Check sheet for the modelled part. Datum: model origin and axes. Units: mm. Face numbers are marked on the shaded views. A direction names the side the tool comes from. Round coordinates to 2 decimals unless told otherwise and drop trailing zeros. Order: outer loops, then holes, each group sorted by start corner. A loop starts at its lowest first (then second) coordinate and runs counter-clockwise, first axis right, second up.
Q1. Cross-section at A-A on z = 9.5. Record the cut outline in (x, y), then the cut area to 3 significant figures.
Q2. Cross-section at B-B on x = 1.8. Record the cut outline in (y, z).
Q3. Cross-section at C-C on y = 8.25. Record the cut outline in (x, z).
Q4. Set-up check for the marked faces 5, 6, 7, 8 and 9: record each of +Z, -Z, +X, -X, +Y, -Y from which the full face is reachable in a straight line by a thin tool's end or side.
Q5. Mould release check, pull along Y, two halves, no side actions. Record for the marked faces 1, 2, 3 and 4: +Y half, -Y half, draft (parallel to the pull), parting line (faces both ways), or undercut.
Q6. Scan lines: probe 1 along Y at (x, z) = (1.9, 10); probe 2 along Z at (x, y) = (2.05, -5.25); probe 3 along Y at (x, z) = (0.2, -6.25). Record each from-to range of solid material in increasing order.
Q7. Depth check by flat-ended pin: P1, Ø1.2, axis at x = 1.5, y = -8.5, coming from the +Z side; P2, Ø0.8, axis at x = 1.5, z = -2, coming from the -Y side; P3, Ø0.8, axis at x = 1.5, y = 3, coming from the +Z side. Enter the tip coordinate at first touch or a pass-through.
from build123d import *

# Parameters (mm, degrees)
BOSS_EXTRUDE1_DEPTH = 2.5


with BuildPart() as part:
    # Sketch2 → Boss-Extrude1 (new body)
    with BuildSketch(Plane(origin=(0, 0, 0), x_dir=(0, 0, -1), z_dir=(1, 0, 0))):
        Polygon((-8.75, 11.25), (11.25, -3.75), (11.25, -6.25), (8.75, -6.25), (8.75, -11.25), (3.75, -11.25), (3.75, -6.25), (1.25, -6.25), (1.25, -3.75), (-11.25, -3.75), (-11.25, 1.25), (-8.75, 1.25), (-8.75, 6.25), (-11.25, 6.25), (-11.25, 11.25), align=None)
    extrude(amount=BOSS_EXTRUDE1_DEPTH)


solid = part.part
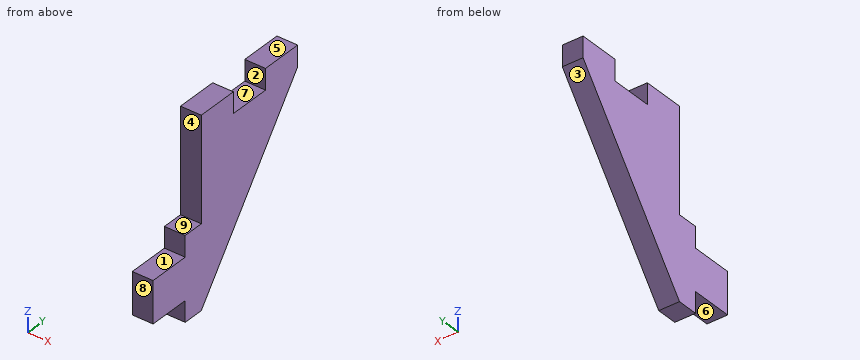
Results found:
1. outline: (0, -3.75) - (2.5, -3.75) - (2.5, 1.25) - (0, 1.25) - close; (0, 6.25) - (2.5, 6.25) - (2.5, 11.25) - (0, 11.25) - close
1. area: 25.0 mm2
2. outline: (-11.25, -8.75) - (-6.25, -8.75) - (-6.25, -11.25) - (-3.75, -11.25) - (11.25, 8.75) - (11.25, 11.25) - (6.25, 11.25) - (6.25, 8.75) - (1.25, 8.75) - (1.25, 11.25) - (-3.75, 11.25) - (-3.75, -1.25) - (-6.25, -1.25) - (-6.25, -3.75) - (-11.25, -3.75) - close
3. outline: (0, 4.75) - (2.5, 4.75) - (2.5, 11.25) - (0, 11.25) - close
4. face 5: +Z, +X, -X, +Y, -Y
4. face 6: -Z, +X, -X, -Y
4. face 7: +Z, +X, -X
4. face 8: +Z, -Z, +X, -X, -Y
4. face 9: +Z, +X, -X, -Y
5. face 1: draft
5. face 2: undercut
5. face 3: +Y half
5. face 4: -Y half
6. probe 1: y = -3.75 to 1.25, 6.25 to 11.25
6. probe 2: z = -11.25 to -1.25
6. probe 3: y = -11.25 to 0
7. P1: stops at z = -3.75
7. P2: stops at y = -6.25
7. P3: stops at z = 8.75
